```python
from build123d import *

# Parameters (mm, degrees)
SKETCH1_W           = 60
SKETCH1_H           = 29
BOSS_EXTRUDE1_DEPTH = 15
SKETCH2_R           = 1.567394172
BOSS_EXTRUDE2_DEPTH = 5
SKETCH3_R           = 1.539361
BOSS_EXTRUDE3_DEPTH = 5


with BuildPart() as part:
    # Sketch1 → Boss-Extrude1 (new body)
    with BuildSketch(Plane(origin=(0, 0, 0), x_dir=(0, 0, -1), z_dir=(1, 0, 0))):
        with Locations((30, 14.5)):
            Rectangle(SKETCH1_W, SKETCH1_H)
    extrude(amount=BOSS_EXTRUDE1_DEPTH)

    # Sketch2 → Boss-Extrude2 (add)
    with BuildSketch(Plane.XY):
        with Locations(Location((3, 24.5, 0), (0, 0, 180))):
            Circle(SKETCH2_R)
        with Locations(Location((3, 14.5, 0), (0, 0, 180))):
            Circle(SKETCH2_R)
        with Locations(Location((3, 4.5, 0), (0, 0, 180))):
            Circle(SKETCH2_R)
    extrude(amount=BOSS_EXTRUDE2_DEPTH)

    # Sketch3 → Boss-Extrude3 (add)
    with BuildSketch(Plane(origin=(0, 0, -60), x_dir=(-1, 0, 0), z_dir=(0, 0, -1))):
        with Locations(Location((-2.947414971, 25.615179296, 0), (0, 0, 180))):
            Circle(SKETCH3_R)
        with Locations(Location((-2.947414971, 3.419179836, 0), (0, 0, 180))):
            Circle(SKETCH3_R)
    extrude(amount=BOSS_EXTRUDE3_DEPTH)


solid = part.part
```
For this review, take the finished solid that the model builds, in its own axes (mm). A direction names the side the tool comes from. Coordinates: 2 decimals unless noted, no trailing zeros. Write each loop counter-clockwise with the first axis right and the second up, starting at its lowest first coordinate (ties: lowest second). Pieces come first, ordered by that corner, then holes.
(1) The part is to be moulded in two halves that separate along Y. For faces 1 (the face through (7, 29, -30)), 2 (the face through (7, 0, -30)), 3 (the face through (3, 26, -65)), 4 (the face through (4.416, 2.957, -62.465)), say which applies: +Y half, -Y half, draft (parallel to the pull), parting line (faces both ways), or undercut.
(2) Add section B-B on x = 13.5. Give the boundary of the cut face in (y, z), then the cut area to 3 significant figures.
(3) Add section A-A on y = 14.5. Give the boundary of the cut face in (x, z).
(4) Add section D-D on y = 8. Give the boundary of the cut face in (x, z), then the cut area to 3 significant figures.
(5) For pin 1 Ø1 at (x, y) = (6, 6) entering from -Z; pin 2 Ø1 at (x, y) = (8.5, 18.5) entering from +Z, all flat-tipped, find the tip position at first contact; note any pin that passes through.
(6) Wall thickness on probe 1 along Z at (x, y) = (13, 11.25); probe 2 along Z at (x, y) = (2.75, 5.5): over which ranges is each line inside the solid? List them lowest first.
(7) Add section C-C on x = 3. Give the boundary of the cut face in (y, z), then the cut area to 3 significant figures.
(8) Tool access review of faces 5 (the face through (2.28, 25.89, 2.46)), 6 (the face through (2.614, 27.118, -62.465)), 7 (the face through (3, 14, 5)): name each direction out of +Z, -Z, +X, -X, +Y, -Y from which nothing blocks a thin tool from reaching the whole face with its end or side.
Answer sheet:
1. face 1: +Y half
1. face 2: -Y half
1. face 3: draft
1. face 4: undercut
2. outline: (0, -60) - (29, -60) - (29, 0) - (0, 0) - close
2. area: 1,740 mm2
3. outline: (0, -60) - (15, -60) - (15, 0) - (4.57, 0) - (4.57, 5) - (1.43, 5) - (1.43, 0) - (0, 0) - close
4. outline: (0, -60) - (15, -60) - (15, 0) - (0, 0) - close
4. area: 900 mm2
5. pin 1: stops at z = -60
5. pin 2: stops at z = 0
6. probe 1: z = -60 to 0
6. probe 2: z = -60 to 5
7. outline: (0, -60) - (1.88, -60) - (1.88, -65) - (4.96, -65) - (4.96, -60) - (24.08, -60) - (24.08, -65) - (27.15, -65) - (27.15, -60) - (29, -60) - (29, 0) - (26.07, 0) - (26.07, 5) - (22.93, 5) - (22.93, 0) - (16.07, 0) - (16.07, 5) - (12.93, 5) - (12.93, 0) - (6.07, 0) - (6.07, 5) - (2.93, 5) - (2.93, 0) - (0, 0) - close
7. area: 1,820 mm2
8. face 5: +Z
8. face 6: -Z
8. face 7: +Z, +X, -X, +Y, -Y
